Source: CAD feature listing. Evaluate the final solid. Frame: model axes, mm. Face numbers are marked on the shaded views. A direction names the side the tool comes from. Give positions to 0.01 mm unless a question says otherwise; leave off trailing zeros. Loops run counter-clockwise (first coordinate to the right, second up) from the corner with the lowest first, then second, coordinate; pieces in that order, holes last. Notation, with made-up numbers: M -37.5,62 L -12.5,62 A19 cw -12.5,77 Z; hole C 30.5,-7 d6. An arc over 180 degrees is marked long. Answer in a Markdown table with one row per item.
```python
from build123d import *

# Parameters (mm, degrees)
PAD_DEPTH            = 30
POCKET_DEPTH         = 25
SKETCH004_W          = 18
SKETCH004_H          = 22.5
PAD001_DEPTH         = 19
SKETCH003_W          = 7.75
SKETCH003_H          = 11.25
POCKET002_DEPTH      = 5
POCKET002_DEPTH_BACK = 24
SKETCH005_W          = 18
SKETCH005_H          = 3.05
PAD002_DEPTH         = 2.73
PAD002_DEPTH_BACK    = 25.23
SKETCH006_W          = 3.5
SKETCH006_H          = 2.5
POCKET003_DEPTH      = 18
SKETCH002_R          = 4
POCKET001_DEPTH      = 35
POCKET001_DEPTH_BACK = 5


with BuildPart() as part:
    # Sketch → Pad (new body)
    with BuildSketch(Plane.XY):
        with BuildLine():
            Line((0, 0), (18, 0))
            ThreePointArc((18, 0), (21.175416, 25), (18, 50))
            Line((18, 50), (0, 50))
            ThreePointArc((0, 50), (-3.175416, 25), (0, 0))
        make_face()
    extrude(amount=-PAD_DEPTH)

    # Sketch001 → Pocket (cut)
    with BuildSketch(Plane.XY):
        with BuildLine():
            Line((3.9, 2.225), (14.2, 2.225))
            ThreePointArc((14.2, 2.225), (18.099995, 25.004308), (14.15, 47.775))
            Line((14.15, 47.775), (3.85, 47.775))
            ThreePointArc((3.85, 47.775), (-0.049995, 24.995692), (3.9, 2.225))
        make_face()
    extrude(amount=-POCKET_DEPTH, mode=Mode.SUBTRACT)

    # Sketch004 → Pad001 (join)
    with BuildSketch(Plane(origin=(0, 0, -30), x_dir=(1, 0, 0), z_dir=(0, 0, -1))):
        with Locations((9, -25)):
            Rectangle(SKETCH004_W, SKETCH004_H)
    extrude(amount=PAD001_DEPTH)

    # Sketch003 (on Face5 of Pocket001) → Pocket002 (cut, two sides)
    with BuildSketch(Plane(origin=(0, 0, -30), x_dir=(1, 0, 0), z_dir=(0, 0, -1))) as pocket002_sk:
        with Locations((5.875, -13.125)):
            Rectangle(SKETCH003_W, SKETCH003_H)
    extrude(amount=-POCKET002_DEPTH, mode=Mode.SUBTRACT)
    extrude(pocket002_sk.sketch, amount=POCKET002_DEPTH_BACK, mode=Mode.SUBTRACT)

    # Sketch005 (on Face11 of Pocket001) → Pad002 (join, two sides)
    with BuildSketch(Plane.XZ.offset(-13.75)) as pad002_sk:
        with Locations((9, -50.475)):
            Rectangle(SKETCH005_W, SKETCH005_H)
    extrude(amount=PAD002_DEPTH)
    extrude(pad002_sk.sketch, amount=-PAD002_DEPTH_BACK)

    # Sketch006 (on Face16 of Pocket001) → Pocket003 (cut)
    with BuildSketch(Plane.YZ.offset(18)):
        with Locations((25, -50.75)):
            Rectangle(SKETCH006_W, SKETCH006_H)
    extrude(amount=-POCKET003_DEPTH, mode=Mode.SUBTRACT)

    # Sketch002 (on Face11 of Pocket) → Pocket001 (cut, two sides)
    with BuildSketch(Plane.XY.offset(-25)) as pocket001_sk:
        with Locations((9.05, 25)):
            Circle(SKETCH002_R)
    extrude(amount=-POCKET001_DEPTH, mode=Mode.SUBTRACT)
    extrude(pocket001_sk.sketch, amount=POCKET001_DEPTH_BACK, mode=Mode.SUBTRACT)


solid = part.part
```
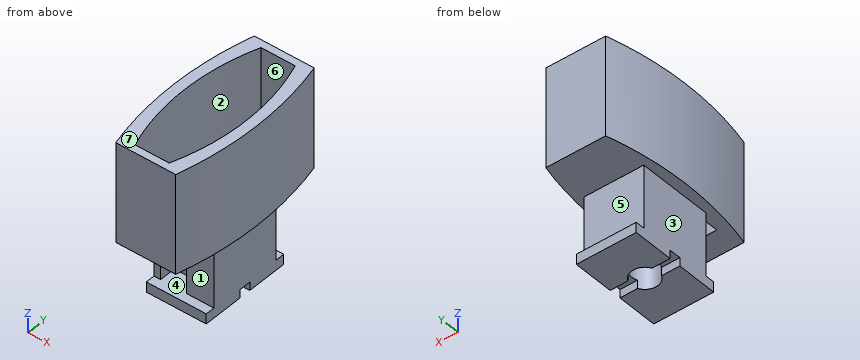
Q1. Contact query for flat-ended pins moving along their axis: pin 1 Ø1 at (y, z) = (12, -43) entering from +X; pin 2 Ø24 at (y, z) = (18.5, -42.5) entering from +X; pin 3 Ø0.6 at (x, z) = (0.5, -40) entering from -Y; pin 4 Ø2 at (x, y) = (6.5, 38) entering from +Z. Output: stop coordinate, or through.
Values follow:
| item | result |
|---|---|
| pin 1 | through |
| pin 2 | x = 18 |
| pin 3 | y = 13.75 |
| pin 4 | z = -25 |
Q2. Reachability of the marked faces 1, 2, 3 and 4 from +Z, -Z, +X, -X, +Y, -Y: full face, straight path, thin tool, end or side. Return the list, or none.
Values follow:
| item | result |
|---|---|
| face 1 | +X, -X, -Y |
| face 2 | +Z |
| face 3 | -Z, -X, +Y, -Y |
| face 4 | -Y |
Q3. Section query D-D (z = -26.5). Output: boundary loops of the cut face in (x, y), plus the area to 3 significant figures.
Values follow:
| item | result |
|---|---|
| outline | M 0,0 L 18,0 A100 ccw 18,50 L 0,50 A100 ccw Z; hole M 2,7.5 L 9.75,7.5 L 9.75,18.75 L 2,18.75 Z; hole C 9.05,25 d8 |
| area | 975 mm^2 |
Q4. Mould query, pull axis Z, two halves, no side actions, for the marked faces 5, 6 and 7. Classes: +Z half, -Z half, draft (parallel to the pull), parting line (faces both ways), or undercut.
Values follow:
| item | result |
|---|---|
| face 5 | undercut |
| face 6 | draft |
| face 7 | +Z half |
Q5. Section query B-B (y = 25). Output: boundary loops of the cut face in (x, z).
Values follow:
| item | result |
|---|---|
| outline | M -3.18,-30 L 0,-30 L 0,-49.5 L 5.05,-49.5 L 5.05,-25 L -0.05,-25 L -0.05,0 L -3.18,0 Z; M 13.05,-49.5 L 18,-49.5 L 18,-30 L 21.18,-30 L 21.18,0 L 18.1,0 L 18.1,-25 L 13.05,-25 Z |
Q6. Section query A-A (x = 9.05). Output: boundary loops of the cut face in (y, z) (3 decimals), plus the area to 3 significant figures.
Values follow:
| item | result |
|---|---|
| outline | M 0,-30 L 7.5,-30 L 7.5,-25 L 2.225,-25 L 2.225,0 L 0,0 Z; M 11.02,-52 L 21,-52 L 21,-25 L 18.75,-25 L 18.75,-48.95 L 11.02,-48.95 Z; M 29,-52 L 38.98,-52 L 38.98,-48.95 L 36.25,-48.95 L 36.25,-30 L 50,-30 L 50,0 L 47.775,0 L 47.775,-25 L 29,-25 Z |
| area | 506 mm^2 |
Q7. Section query C-C (z = -35). Output: boundary loops of the cut face in (x, y).
Values follow:
| item | result |
|---|---|
| outline | M 0,13.75 L 2,13.75 L 2,18.75 L 9.75,18.75 L 9.75,13.75 L 18,13.75 L 18,36.25 L 0,36.25 Z; hole C 9.05,25 d8 |
Q8. Ray query, probe 1 along X at (y, z) = (25, -38.5); probe 2 along X at (y, z) = (24.5, -13); probe 3 along Y at (x, z) = (7.5, -22.5) (3 decimals). Return the intervals inside material, ascending. Write a range as from..to.
Values follow:
| item | result |
|---|---|
| probe 1 | 0..5.05, 13.05..18 |
| probe 2 | -3.17..-0.05, 18.1..21.17 |
| probe 3 | 0..2.225, 47.775..50 |
